Can you work these out from the drawing? Everything is in mm from the part's minimum corner. A direction names the side the tool comes from. Give positions to 0.01 mm unless a question says otherwise; leave off trailing zeros. Write each loop counter-clockwise with the first axis right and the second up, starting at its lowest first coordinate (ties: lowest second). Pieces come first, ordered by that corner, then holes. Notation, with made-up numbers: (62.5, 85) -> (102.5, 85) arc R34 ccw to (102.5, 115) -> close; hole circle Ø2 at (-35.5, 40). An arc over 180 degrees is marked (long way). Answer as CSV lines item,"result". Start each with the question number.
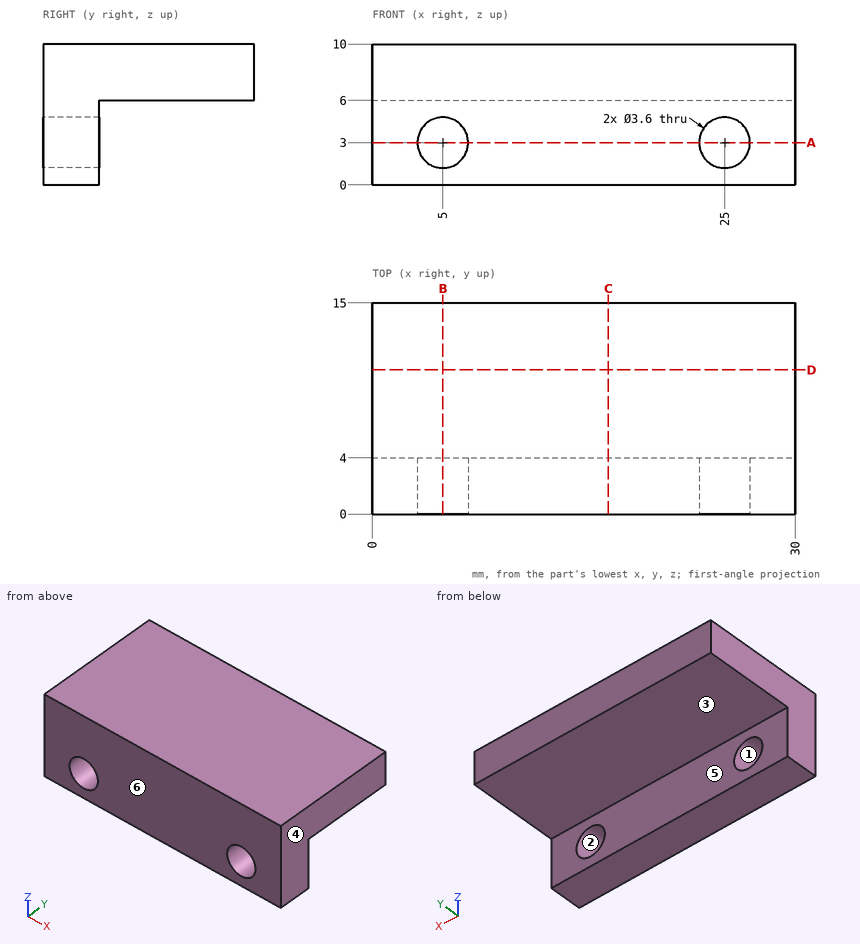
Item 1: If we section it at B-B (x = 5): Please give me the cut outline in (y, z), and give its area (3 significant figures).
Item 2: We'd pull the mould along Z, two halves only. Please class the marked faces 1, 2, 3 and 4: released by +Z, released by -Z, zero draft, split by the parting line, or undercut.
Item 3: If we section it at C-C (x = 16.75): Please give me the cut outline in (y, z).
Item 4: If we section it at A-A (z = 3): Please give me the cut outline in (x, y).
Item 5: If we section it at D-D (y = 10.25): Please give me the cut outline in (x, z), and give its area (3 significant figures).
Item 6: If I drill on line 1 (X direction, y = 2.7, z = 3); line 2 (Z direction, x = 5, y = 2.05); line 3 (Y direction, x = 16.75, z = 5.75), over which ranges is the centre line in solid material (lowest first)? Write a range as [from, to].
Item 7: For the marked faces 5 and 6, which set-ups out of +Z, -Z, +X, -X, +Y, -Y let a thin tool reach every point of the face, with its end or its side?
Item 8: I'm going to push flat-ended pins straight in: pin 1 (5 mm diameter, centred on x = 21.5, z = 4, fed in from +Y); pin 2 (3 mm diameter, centred on x = 25.5, y = 6, fed in from -Z); pin 3 (2 mm diameter, centred on x = 5, z = 3, fed in from -Y); pin 4 (3 mm diameter, centred on x = 14, z = 1, fed in from +Y). Where does each tip first touch, or does it pass through?
Final values:
1,outline,"(0, 0) -> (4, 0) -> (4, 1.2) -> (0, 1.2) -> close; (0, 4.8) -> (4, 4.8) -> (4, 6) -> (15, 6) -> (15, 10) -> (0, 10) -> close"
1,area,"69.6 mm2"
2,face 1,"undercut"
2,face 2,"undercut"
2,face 3,"released by -Z"
2,face 4,"zero draft"
3,outline,"(0, 0) -> (4, 0) -> (4, 6) -> (15, 6) -> (15, 10) -> (0, 10) -> close"
4,outline,"(0, 0) -> (3.2, 0) -> (3.2, 4) -> (0, 4) -> close; (6.8, 0) -> (23.2, 0) -> (23.2, 4) -> (6.8, 4) -> close; (26.8, 0) -> (30, 0) -> (30, 4) -> (26.8, 4) -> close"
5,outline,"(0, 6) -> (30, 6) -> (30, 10) -> (0, 10) -> close"
5,area,"120 mm2"
6,line 1,"[0, 3.2], [6.8, 23.2], [26.8, 30]"
6,line 2,"[0, 1.2], [4.8, 10]"
6,line 3,"[0, 4]"
7,face 5,"-Z, +X, -X, +Y"
7,face 6,"+Z, -Z, +X, -X, -Y"
8,pin 1,"y = 15"
8,pin 2,"z = 6"
8,pin 3,"through"
8,pin 4,"y = 4"
